Can you work these out from the drawing? Everything is in mm from the part's minimum corner. A direction names the side the tool comes from. Round coordinates to 2 decimals unless told otherwise and drop trailing zeros. Write each loop counter-clockwise with the first axis right and the second up, starting at its lowest first coordinate (ties: lowest second). Pieces come first, ordered by that corner, then holes. Notation, with made-up numbers: (-8, 72) -> (44, 72) arc R22 cw to (44, 100) -> close; hole circle Ø4 at (32.25, -38). An arc over 180 degrees is marked (long way). Put each result on its own line as item: value. Start each with the question number.
1. Suppose I cut it at D-D (x = 32.5). Please give me the cut outline in (y, z).
2. Which directions (+Z, -Z, +X, -X, +Y, -Y) give clear straight access to the entire face, cutting with the end or side of a thin tool? Please do the marked faces 1, 2 and 3.
3. Suppose I cut it at B-B (z = 49.5). Please give me the cut outline in (x, y) (3 decimals).
4. We'd pull the mould along Z, two halves only. Please class the marked faces 4, 5, 6 and 7: +Z half, -Z half, draft (parallel to the pull), parting line (faces both ways), or undercut.
5. Suppose I cut it at A-A (y = 2.5). Please give me the cut outline in (x, z) (3 decimals).
6. I need wall thicknesses on probe 1 along Z at (x, y) = (12.5, 4.25); probe 2 along Z at (x, y) = (16.5, 6.25); probe 3 along X at (y, z) = (2.25, 47) (3 decimals). Which ranges of each line are inside material? Lowest first, please. Write a range as from..to.
7. Suppose I cut it at C-C (z = 30.5). Please give me the cut outline in (x, y), then the cut area to 3 significant figures.
8. For pin 1 (1.9 mm diameter, centred on y = 4, z = 48.5, fed in from +X) (3 decimals); pin 2 (1 mm diameter, centred on y = 4, z = 44.5, fed in from -X) (3 decimals); pin 3 (1.5 mm diameter, centred on x = 19.5, y = 3, fed in from +Z); pin 4 (3 mm diameter, centred on x = 21.5, y = 3.5, fed in from +Z), each with a flat end and sliding along its axis, tell me the tip position at first contact or that it passes through.
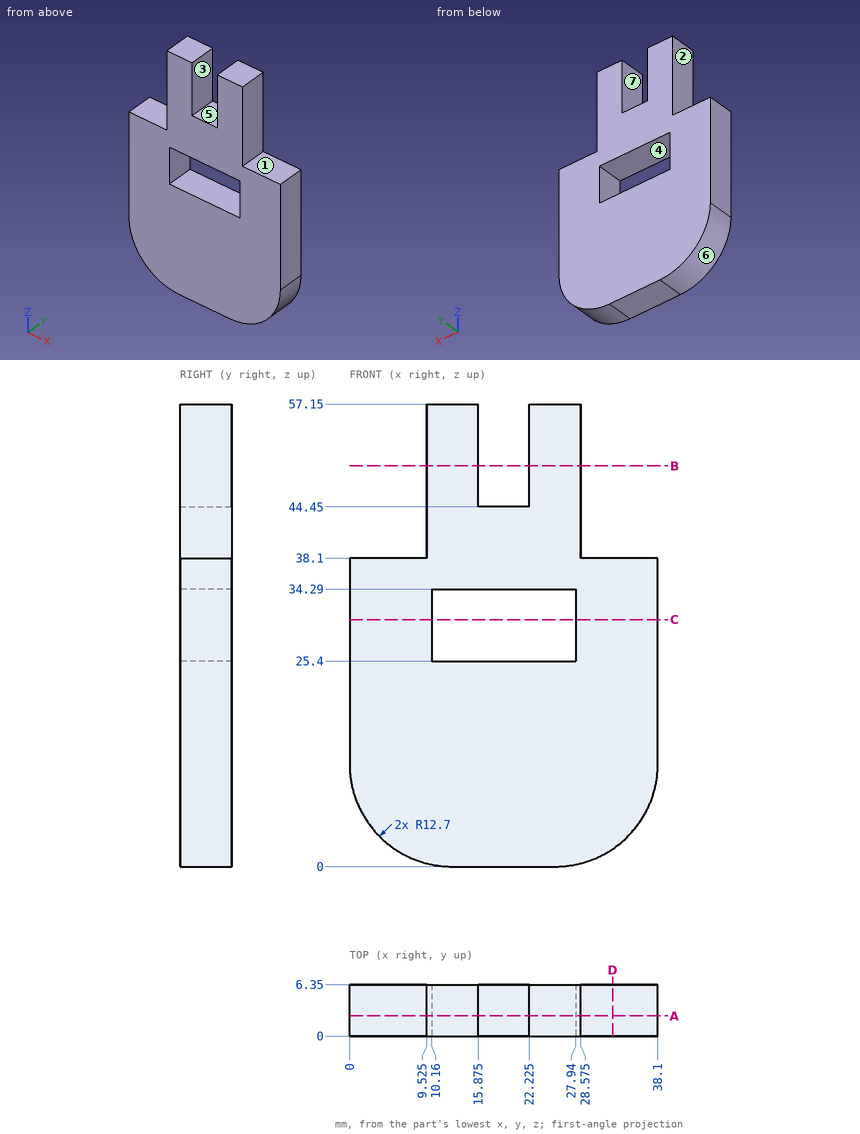
Verdict:
1. outline: (0, 2.17) -> (6.35, 2.17) -> (6.35, 38.1) -> (0, 38.1) -> close
2. face 1: +Z, +X, +Y, -Y
2. face 2: +Z, -X, +Y, -Y
2. face 3: +Z, +Y, -Y
3. outline: (9.525, 0) -> (15.875, 0) -> (15.875, 6.35) -> (9.525, 6.35) -> close; (22.225, 0) -> (28.575, 0) -> (28.575, 6.35) -> (22.225, 6.35) -> close
4. face 4: undercut
4. face 5: +Z half
4. face 6: -Z half
4. face 7: draft
5. outline: (0, 12.7) arc R12.7 ccw to (12.7, 0) -> (25.4, 0) arc R12.7 ccw to (38.1, 12.7) -> (38.1, 38.1) -> (28.575, 38.1) -> (28.575, 57.15) -> (22.225, 57.15) -> (22.225, 44.45) -> (15.875, 44.45) -> (15.875, 57.15) -> (9.525, 57.15) -> (9.525, 38.1) -> (0, 38.1) -> close; hole (10.16, 25.4) -> (27.94, 25.4) -> (27.94, 34.29) -> (10.16, 34.29) -> close
6. probe 1: z = 0..25.4, 34.29..57.15
6. probe 2: z = 0..25.4, 34.29..44.45
6. probe 3: x = 9.525..15.875, 22.225..28.575
7. outline: (0, 0) -> (10.16, 0) -> (10.16, 6.35) -> (0, 6.35) -> close; (27.94, 0) -> (38.1, 0) -> (38.1, 6.35) -> (27.94, 6.35) -> close
7. area: 129 mm^2
8. pin 1: stops at x = 28.575
8. pin 2: stops at x = 9.525
8. pin 3: stops at z = 44.45
8. pin 4: stops at z = 57.15
